The drawing under review shows one solid part. Ordinate dimensions are in mm from its lowest x, y, z. Coordinates: 2 decimals unless noted, no trailing zeros. Loops run counter-clockwise (first coordinate to the right, second up) from the corner with the lowest first, then second, coordinate; pieces in that order, holes last. Notation, with made-up numbers: M 20,-15.5 L 50,-15.5 A7 ccw 50,-9.5 Z; hole C 24.5,33.25 d10. An arc over 180 degrees is marked long. Use one line per item in the form item = value.
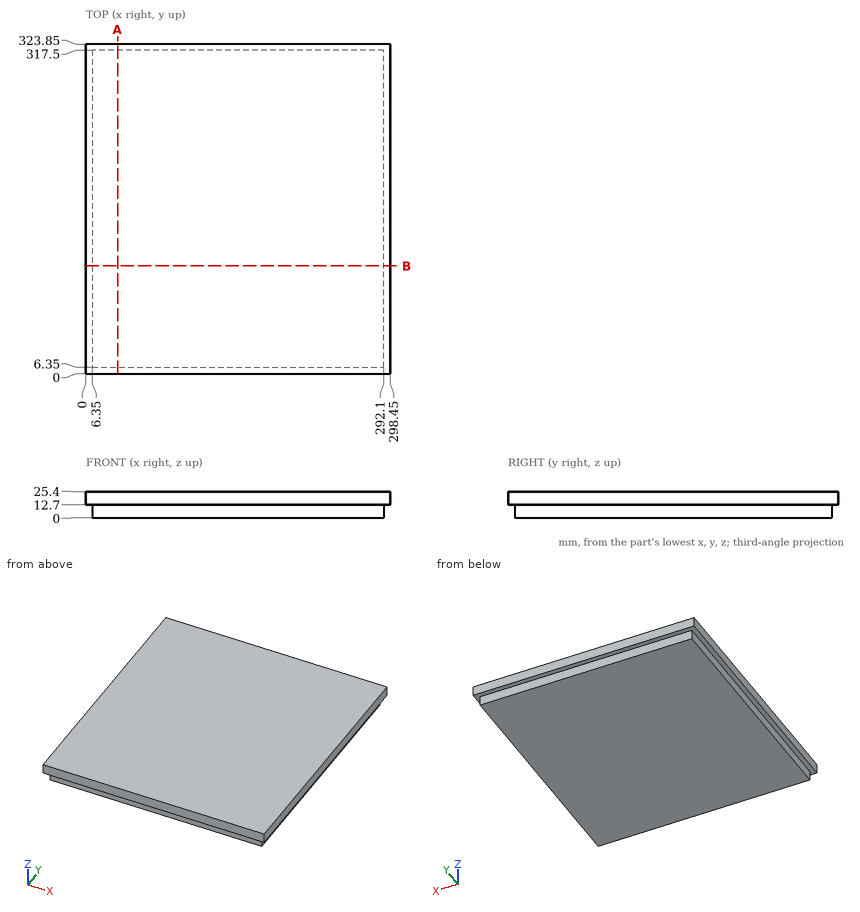
1. Wall thickness on line 1 along Y through (x, z) = (58, 4); line 2 along X through (y, z) = (113, 6.75): over which ranges is each line inside the solid? List them lowest first. Write a range as from..to.
Computed values:
line_1 = 6.35..317.5
line_2 = 6.35..292.1
2. For pin 1 Ø4 at (x, z) = (218.5, 8.5) entering from -Y; pin 2 Ø2 at (x, y) = (139.5, 76.5) entering from -Z; pin 3 Ø14 at (y, z) = (199, 4.5) entering from -X; pin 4 Ø10 at (y, z) = (114.5, 4.5) entering from +X, all flat-tipped, find the tip position at first contact; note any pin that passes through.
Computed values:
pin_1 = 6.35
pin_2 = 0
pin_3 = 6.35
pin_4 = 292.1
3. Consider section A-A on x = 31. Write out the cut boundary in (y, z).
Computed values:
outline = M 0,12.7 L 6.35,12.7 L 6.35,0 L 317.5,0 L 317.5,12.7 L 323.85,12.7 L 323.85,25.4 L 0,25.4 Z
4. Consider section B-B on y = 106. Write out the cut boundary in (x, z).
Computed values:
outline = M 0,12.7 L 6.35,12.7 L 6.35,0 L 292.1,0 L 292.1,12.7 L 298.45,12.7 L 298.45,25.4 L 0,25.4 Z
